Here's how the part is built. I have some questions about the finished solid (model axes, mm). A direction names the side the tool comes from. Coordinates: 2 decimals unless noted, no trailing zeros. Write each loop counter-clockwise with the first axis right and the second up, starting at its lowest first coordinate (ties: lowest second). Pieces come first, ordered by that corner, then holes. Notation, with made-up numbers: M 56.25,50 L 65.25,50 A24 ccw 65.25,82 Z; hole C 20,86.5 d11. An arc over 180 degrees is marked long. Write each question's results on one line, items separated by ' | '. Start each with the question number.
from build123d import *

# Parameters (mm, degrees)
SKETCH1_W           = 125
SKETCH1_H           = 190
SKETCH1_R           = 2.5
SKETCH1_R_2         = 1.75
BOSS_EXTRUDE1_DEPTH = 3
CUT_EXTRUDE1_START  = 2
SKETCH1_3_R         = 2.5
SKETCH1_3_R_2       = 1.75
CUT_EXTRUDE1_DEPTH  = 1
SKETCH2_W           = 30
SKETCH2_H           = 130
CUT_EXTRUDE2_DEPTH  = 114.75521966
FILLET1_R           = 20
FILLET2_R           = 10
BOSS_EXTRUDE2_DEPTH = 3


with BuildPart() as part:
    # Sketch1 → Boss-Extrude1 (new body)
    # profile 1 of 5: a face of its own
    with BuildSketch(Plane(origin=(0, 0, 0), x_dir=(1, 0, 0), z_dir=(0, 1, 0))):
        Rectangle(SKETCH1_W, SKETCH1_H)
        with Locations((-12, 55.5)):
            Circle(SKETCH1_R, mode=Mode.SUBTRACT)
        with Locations((12, 55.5)):
            Circle(SKETCH1_R, mode=Mode.SUBTRACT)
        with Locations((-12, -55)):
            Circle(SKETCH1_R, mode=Mode.SUBTRACT)
        with Locations((12, -55)):
            Circle(SKETCH1_R, mode=Mode.SUBTRACT)
    # profile 2 of 5: a face of its own
    with BuildSketch(Plane(origin=(0, 0, 0), x_dir=(1, 0, 0), z_dir=(0, 1, 0))):
        with Locations((-12, -55)):
            Circle(SKETCH1_R)
        with Locations(Location((-12, -55, 0), (0, 0, 270))):
            Circle(SKETCH1_R_2, mode=Mode.SUBTRACT)
    # profile 3 of 5: a face of its own
    with BuildSketch(Plane(origin=(0, 0, 0), x_dir=(1, 0, 0), z_dir=(0, 1, 0))):
        with Locations((12, -55)):
            Circle(SKETCH1_R)
        with Locations(Location((12, -55, 0), (0, 0, 270))):
            Circle(SKETCH1_R_2, mode=Mode.SUBTRACT)
    # profile 4 of 5: a face of its own
    with BuildSketch(Plane(origin=(0, 0, 0), x_dir=(1, 0, 0), z_dir=(0, 1, 0))):
        with Locations((12, 55.5)):
            Circle(SKETCH1_R)
        with Locations(Location((12, 55.5, 0), (0, 0, 270))):
            Circle(SKETCH1_R_2, mode=Mode.SUBTRACT)
    # profile 5 of 5: a face of its own
    with BuildSketch(Plane(origin=(0, 0, 0), x_dir=(1, 0, 0), z_dir=(0, 1, 0))):
        with Locations((-12, 55.5)):
            Circle(SKETCH1_R)
        with Locations(Location((-12, 55.5, 0), (0, 0, 270))):
            Circle(SKETCH1_R_2, mode=Mode.SUBTRACT)
    extrude(amount=BOSS_EXTRUDE1_DEPTH)

    # Sketch1<3> → Cut-Extrude1 (cut)
    # profile 1 of 4: a face of its own
    with BuildSketch(Plane(origin=(0, 0, 0), x_dir=(1, 0, 0), z_dir=(0, 1, 0)).offset(CUT_EXTRUDE1_START)):
        with Locations(Location((-12, -55, 0), (0, 0, 270))):
            Circle(SKETCH1_3_R)
        with Locations(Location((-12, -55, 0), (0, 0, 270))):
            Circle(SKETCH1_3_R_2, mode=Mode.SUBTRACT)
    # profile 2 of 4: a face of its own
    with BuildSketch(Plane(origin=(0, 0, 0), x_dir=(1, 0, 0), z_dir=(0, 1, 0)).offset(CUT_EXTRUDE1_START)):
        with Locations(Location((12, 55.5, 0), (0, 0, 270))):
            Circle(SKETCH1_3_R)
        with Locations(Location((12, 55.5, 0), (0, 0, 270))):
            Circle(SKETCH1_3_R_2, mode=Mode.SUBTRACT)
    # profile 3 of 4: a face of its own
    with BuildSketch(Plane(origin=(0, 0, 0), x_dir=(1, 0, 0), z_dir=(0, 1, 0)).offset(CUT_EXTRUDE1_START)):
        with Locations(Location((-12, 55.5, 0), (0, 0, 270))):
            Circle(SKETCH1_3_R)
        with Locations(Location((-12, 55.5, 0), (0, 0, 270))):
            Circle(SKETCH1_3_R_2, mode=Mode.SUBTRACT)
    # profile 4 of 4: a face of its own
    with BuildSketch(Plane(origin=(0, 0, 0), x_dir=(1, 0, 0), z_dir=(0, 1, 0)).offset(CUT_EXTRUDE1_START)):
        with Locations(Location((12, -55, 0), (0, 0, 270))):
            Circle(SKETCH1_3_R)
        with Locations(Location((12, -55, 0), (0, 0, 270))):
            Circle(SKETCH1_3_R_2, mode=Mode.SUBTRACT)
    extrude(amount=CUT_EXTRUDE1_DEPTH, mode=Mode.SUBTRACT)

    # Sketch2 → Cut-Extrude2 (cut, through all)
    with BuildSketch(Plane(origin=(0, 3, 0), x_dir=(1, 0, 0), z_dir=(0, 1, 0))):
        with Locations((47.5, 0)):
            Rectangle(SKETCH2_W, SKETCH2_H)
        with Locations((-47.5, 0)):
            Rectangle(SKETCH2_W, SKETCH2_H)
    extrude(amount=-CUT_EXTRUDE2_DEPTH, mode=Mode.SUBTRACT)

    # Fillet1
    fillet1_edges = [part.edges().sort_by_distance(p)[0] for p in [
        (32.5, 1.5, 65),
        (32.5, 1.5, -65),
        (-32.5, 1.5, -65),
        (-32.5, 1.5, 65),
    ]]
    fillet(fillet1_edges, radius=FILLET1_R)

    # Fillet2
    fillet2_edges = [part.edges().sort_by_distance(p)[0] for p in [
        (-62.5, 1.5, 95),
        (-62.5, 1.5, -95),
        (62.5, 1.5, -95),
        (62.5, 1.5, 95),
    ]]
    fillet(fillet2_edges, radius=FILLET2_R)

    # Sketch3 → Boss-Extrude2 (add)
    with BuildSketch(Plane(origin=(0, 3, 0), x_dir=(1, 0, 0), z_dir=(0, 1, 0))):
        with BuildLine():
            Line((-59.5, 68), (-62.5, 68))
            Line((-62.5, 68), (-62.5, 65))
            Line((-62.5, 65), (-52.5, 65))
            ThreePointArc((-52.5, 65), (-38.357864376, 59.142135624), (-32.5, 45))
            Line((-32.5, 45), (-32.5, -45))
            ThreePointArc((-32.5, -45), (-38.357864376, -59.142135624), (-52.5, -65))
            Line((-52.5, -65), (-62.5, -65))
            Line((-62.5, -65), (-62.5, -68))
            Line((-62.5, -68), (-59.5, -68))
            Line((-59.5, -68), (-52.5, -68))
            ThreePointArc((-52.5, -68), (-36.236544033, -61.263455967), (-29.5, -45))
            Line((-29.5, -45), (-29.5, 45))
            ThreePointArc((-29.5, 45), (-36.236544033, 61.263455967), (-52.5, 68))
            Line((-52.5, 68), (-59.5, 68))
        make_face()
        with BuildLine():
            Line((59.5, 68), (62.5, 68))
            Line((62.5, 68), (62.5, 65))
            Line((62.5, 65), (52.5, 65))
            ThreePointArc((52.5, 65), (38.357864376, 59.142135624), (32.5, 45))
            Line((32.5, 45), (32.5, -45))
            ThreePointArc((32.5, -45), (38.357864376, -59.142135624), (52.5, -65))
            Line((52.5, -65), (62.5, -65))
            Line((62.5, -65), (62.5, -68))
            Line((62.5, -68), (59.5, -68))
            Line((59.5, -68), (52.5, -68))
            ThreePointArc((52.5, -68), (36.236544033, -61.263455967), (29.5, -45))
            Line((29.5, -45), (29.5, 45))
            ThreePointArc((29.5, 45), (36.236544033, 61.263455967), (52.5, 68))
            Line((52.5, 68), (59.5, 68))
        make_face()
        with BuildLine():
            Line((-52.5, -92), (-59.641428429, -92))
            ThreePointArc((-59.641428429, -92), (-56.372983346, -94.219544457), (-52.5, -95))
            Line((-52.5, -95), (52.5, -95))
            ThreePointArc((52.5, -95), (56.372983346, -94.219544457), (59.641428429, -92))
            Line((59.641428429, -92), (52.5, -92))
            Line((52.5, -92), (-52.5, -92))
        make_face()
        with BuildLine():
            Line((-52.5, 92), (-59.641428429, 92))
            ThreePointArc((-59.641428429, 92), (-56.372983346, 94.219544457), (-52.5, 95))
            Line((-52.5, 95), (52.5, 95))
            ThreePointArc((52.5, 95), (56.372983346, 94.219544457), (59.641428429, 92))
            Line((59.641428429, 92), (52.5, 92))
            Line((52.5, 92), (-52.5, 92))
        make_face()
    extrude(amount=BOSS_EXTRUDE2_DEPTH)


solid = part.part
1) I want a section at D-D, the plane x = 19. Write out the boundary of the cut face in (y, z).
2) For pin 1 Ø1.5 at (x, y) = (-55.5, 4.5) entering from -Z; pin 2 Ø1 at (y, z) = (3, 51) entering from +X; pin 3 Ø3 at (x, y) = (-59, 3.5) entering from -Z, each with a flat end and sliding along its axis, tell me the tip position at first contact or that it passes through.
3) I want a section at B-B, the plane y = 4.5. Give the number of separate pieces and of enclosed holes in the cut face, then the cut area to 3 significant figures.
4) I want a section at A-A, the plane x = 47. Write out the boundary of the cut face in (y, z).
5) Please list where these lines run through material, in increasing order: line 1 (X direction, y = 3.55, z = 16); line 2 (X direction, y = 2.7, z = 55); line 3 (X direction, y = 2.6, z = -55.5). Write a range as [from, to].
6) I want a section at C-C, the plane z = 7. Write out the boundary of the cut face in (x, y), then the cut area to 3 significant figures.
7) We'd pull the mould along Z, two halves only. Please class faces 1 (the flat face through (-62.5, 2, 75)), 2 (the cylindrical face through (-11.474, 0.986, -53.831)), 3 (the flat face through (-1, 3, -95)), 4 (the flat face through (14, 2, -55)): pulls with the +Z half, pulls with the -Z half, needs draft (parallel to the pull), parting line crosses it, or undercut.
8) For faces 5 (the flat face through (-1, 3, 95)), 6 (the cylindrical face through (12.526, 0.986, 56.669)), 7 (the flat face through (-58, 3, -65)), 8 (the flat face through (57, 3, -65)), 9 (the cylindrical face through (36.416, 4.479, 61.441)), which set-ups out of +Z, -Z, +X, -X, +Y, -Y let a thin tool reach every point of the face, with its end or its side?
Output:
1) outline: M 0,-95 L 6,-95 L 6,-92 L 3,-92 L 3,92 L 6,92 L 6,95 L 0,95 Z
2) pin 1: stops at z = -94.74 | pin 2: stops at x = 33.59 | pin 3: stops at z = -93.66
3) separate pieces: 4 | enclosed holes: 0 | area: 1,750 mm2
4) outline: M 0,-95 L 6,-95 L 6,-92 L 3,-92 L 3,-67.33 L 6,-67.33 L 6,-64.23 L 0,-64.23 Z; M 0,64.23 L 6,64.23 L 6,67.33 L 3,67.33 L 3,92 L 6,92 L 6,95 L 0,95 Z
5) line 1: x = [-32.5, -29.5], [29.5, 32.5] | line 2: x = [-35.18, -14.5], [-9.5, 9.5], [14.5, 35.18] | line 3: x = [-35.48, -14.5], [-9.5, 9.5], [14.5, 35.48]
6) outline: M -32.5,0 L 32.5,0 L 32.5,6 L 29.5,6 L 29.5,3 L -29.5,3 L -29.5,6 L -32.5,6 Z | area: 213 mm2
7) face 1: needs draft | face 2: undercut | face 3: pulls with the -Z half | face 4: undercut
8) face 5: +Z, +X, -X, +Y, -Y | face 6: +Y, -Y | face 7: -X, +Y, -Y | face 8: +X, +Y, -Y | face 9: +Y
